Model file for the job. Use its own axes, mm. Give positions to 0.01 mm unless a question says otherwise; leave off trailing zeros. Order: outer loops, then holes, each group sorted by start corner. A loop starts at its lowest first (then second) coordinate and runs counter-clockwise, first axis right, second up. Notation, with made-up numbers: (79.25, 9) -> (111.25, 9) arc R22 cw to (111.25, 48) -> close; hole circle Ø6 at (30.5, -2). An arc over 180 degrees is marked (long way). Use CSV: the item, a comma, the result in double quotes. Start each with the question number.
1. Drop a flat-ended pin along its axis: pin 1 (0.9 mm diameter, centred on x = 0, y = 2, fed in from +Z). Give the stop position or say it passes through.
2. Cut at B-B on z = -115.9. List the corners of the cut face in (x, y).
3. Cut at A-A on z = -30.5. List the corners of the cut face in (x, y).
4. Wall check: line 1 (Y direction, x = 0.6, z = -115.9); line 2 (Y direction, x = 0.85, z = -21.2); line 3 (Z direction, x = -0.6, y = 150.8). Give the ranges that are in metal, low to high. Write a range as from..to.
5. Cut at C-C on x = 0.75. Give the number of separate pieces and of enclosed holes in the cut face, then the cut area to 3 significant figures.
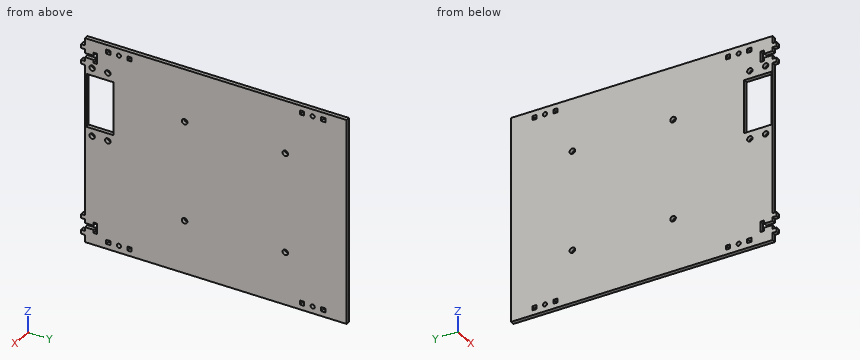
```python
from build123d import *

# Parameters (mm, degrees)
BOSS_EXTRUDE2_DEPTH      = 1.5
BOSS_EXTRUDE2_DEPTH_BACK = 1.5
SKETCH1_R                = 1.575
SKETCH1_R_2              = 2.05
SKETCH1_R_3              = 2.1
SKETCH1_W                = 40.5
SKETCH1_H                = 20.499999995
SKETCH1_W_2              = 3.15
SKETCH1_H_2              = 3.15


with BuildPart() as part:
    # Sketch1 → Boss-Extrude2 (new, two sides: drawn at the far end of the back side and taken through both)
    with BuildSketch(Plane(origin=(0, 0, 0), x_dir=(0, 0, -1), z_dir=(1, 0, 0)).offset(-BOSS_EXTRUDE2_DEPTH_BACK)):
        Polygon((11.425, 0), (8.5, 0), (8.5, -3), (5.5, -3), (5.5, 0), (0, 0), (0, 197), (156, 197), (156, 0), (150.5, 0), (150.5, -3), (147.5, -3), (147.5, 0), (144.575, 0), (144.575, 6.5), (147, 6.5), (147, 9), (139, 9), (139, 6.5), (141.425, 6.5), (141.425, 0), (138.5, 0), (138.5, -3), (135.5, -3), (135.5, 0), (20.5, 0), (20.5, -3), (17.5, -3), (17.5, 0), (14.575, 0), (14.575, 6.5), (17, 6.5), (17, 9), (9, 9), (9, 6.5), (11.425, 6.5), align=None)
        with Locations((5.25, 25.575)):
            Circle(SKETCH1_R, mode=Mode.SUBTRACT)
        with Locations(Location((5.25, 171.425, 0), (0, 0, 180))):
            Circle(SKETCH1_R, mode=Mode.SUBTRACT)
        with Locations((150.75, 171.425)):
            Circle(SKETCH1_R, mode=Mode.SUBTRACT)
        with Locations(Location((150.75, 25.575, 0), (0, 0, 180))):
            Circle(SKETCH1_R, mode=Mode.SUBTRACT)
        with Locations((73.2, 5.35)):
            Circle(SKETCH1_R_2, mode=Mode.SUBTRACT)
        with Locations((73.2, 17.149999995)):
            Circle(SKETCH1_R_2, mode=Mode.SUBTRACT)
        with Locations((21.2, 5.35)):
            Circle(SKETCH1_R_2, mode=Mode.SUBTRACT)
        with Locations((21.2, 17.149999995)):
            Circle(SKETCH1_R_2, mode=Mode.SUBTRACT)
        with Locations((40.1, 75)):
            Circle(SKETCH1_R_3, mode=Mode.SUBTRACT)
        with Locations((40.1, 150.8)):
            Circle(SKETCH1_R_3, mode=Mode.SUBTRACT)
        with Locations(Location((115.9, 75, 0), (0, 0, 180))):
            Circle(SKETCH1_R_3, mode=Mode.SUBTRACT)
        with Locations(Location((115.9, 150.8, 0), (0, 0, 180))):
            Circle(SKETCH1_R_3, mode=Mode.SUBTRACT)
        with Locations((47.2, 11.249999997)):
            Rectangle(SKETCH1_W, SKETCH1_H, mode=Mode.SUBTRACT)
        with Locations((5.25, 17.575)):
            Rectangle(SKETCH1_W_2, SKETCH1_H_2, mode=Mode.SUBTRACT)
        with Locations((5.25, 33.575)):
            Rectangle(SKETCH1_W_2, SKETCH1_H_2, mode=Mode.SUBTRACT)
        with Locations((5.25, 163.425)):
            Rectangle(SKETCH1_W_2, SKETCH1_H_2, mode=Mode.SUBTRACT)
        with Locations((5.25, 179.425)):
            Rectangle(SKETCH1_W_2, SKETCH1_H_2, mode=Mode.SUBTRACT)
        with Locations((150.75, 179.425)):
            Rectangle(SKETCH1_W_2, SKETCH1_H_2, mode=Mode.SUBTRACT)
        with Locations((150.75, 163.425)):
            Rectangle(SKETCH1_W_2, SKETCH1_H_2, mode=Mode.SUBTRACT)
        with Locations((150.75, 33.575)):
            Rectangle(SKETCH1_W_2, SKETCH1_H_2, mode=Mode.SUBTRACT)
        with Locations((150.75, 17.575)):
            Rectangle(SKETCH1_W_2, SKETCH1_H_2, mode=Mode.SUBTRACT)
    extrude(amount=BOSS_EXTRUDE2_DEPTH + BOSS_EXTRUDE2_DEPTH_BACK)


solid = part.part
```
Verdict:
1,pin 1,"z = 0"
2,outline,"(-1.5, 0) -> (1.5, 0) -> (1.5, 72.9) -> (-1.5, 72.9) -> close; (-1.5, 77.1) -> (1.5, 77.1) -> (1.5, 148.7) -> (-1.5, 148.7) -> close; (-1.5, 152.9) -> (1.5, 152.9) -> (1.5, 197) -> (-1.5, 197) -> close"
3,outline,"(-1.5, 0) -> (1.5, 0) -> (1.5, 1) -> (-1.5, 1) -> close; (-1.5, 21.5) -> (1.5, 21.5) -> (1.5, 197) -> (-1.5, 197) -> close"
4,line 1,"0..72.9, 77.1..148.7, 152.9..197"
4,line 2,"0..3.3, 7.4..15.1, 19.2..197"
4,line 3,"-156..-118, -113.8..-42.2, -38..0"
5,separate pieces,"1"
5,enclosed holes,"21"
5,area,"29,600 mm^2"
